Could you check a few things on this model? Use its own coordinates, in mm. A direction names the side the tool comes from. Give positions to 0.01 mm unless a question says otherwise; leave off trailing zeros. Order: outer loops, then holes, each group sorted by start corner. A loop starts at its lowest first (then second) coordinate and runs counter-clockwise, first axis right, second up.
(1) Imagine slicing it at B-B, the plane z = 15.25. Write out the boundary of the cut face in (x, y), then the cut area to 3 significant figures.
(2) On a 3-axis mill with a long thin cutter (end or side, diameter ignored), from which of +Z, -Z, +X, -X, +Y, -Y can I reach the whole of each face in a straight line? I mean faces 1 (the flat face through (85.725, -9, 5)), 2 (the flat face through (85.725, 9, 5)), 3 (the flat face through (95, 9, 5)). Say none if no direction works.
(3) If we mould it in two halves opening along Y, with no side actions, what happens to faces 4 (the cylindrical face through (95.19, 7.14, 2.46)), 5 (the cylindrical face through (42.452, 0.088, 15.16)), 6 (the flat face through (-85.725, 9, 5))? For each: released by +Y, released by -Y, zero draft, split by the parting line, or undercut.
(4) Imagine slicing it at C-C, the plane x = -49. Write out the boundary of the cut face in (y, z) (3 decimals).
(5) Will these pins go through, and if not, where does the flat tip stop? pin 1 (6 mm diameter, centred on y = -2.5, z = 5, fed in from -X); pin 2 (10 mm diameter, centred on y = 5.5, z = 17.5, fed in from -X); pin 3 (5 mm diameter, centred on x = -46.5, z = 5, fed in from -Y); pin 4 (3 mm diameter, centred on x = -93.66, y = -7.62, fed in from -Z).
(6) Imagine slicing it at A-A, the plane z = 7.75. Write out the boundary of the cut face in (x, y) (1 decimal).
(7) If I drill on probe 1 along X at (y, z) = (7.62, 1.45) (1 decimal); probe 2 along X at (y, z) = (-10, 1.75) (3 decimals); probe 3 along X at (y, z) = (0.25, 13.75), over which ranges is the centre line in solid material (lowest first)?
from build123d import *

# Parameters (mm, degrees)
F1_DEPTH = 9.525
F2_R     = 2.8
F3_DEPTH = 9.525
F4_R     = 2
F5_DEPTH = 12.7
F6_SIZE  = 1.27
F7_R     = 5.08
F8_R     = 2.8
F8_R_2   = 1.6
F9_DEPTH = 5


# Not quite as in the source:
# - a length typed as a fraction of an inch, garbled in the dataset ("3 / 203.2 mm" for 3/8 in), is restored


with BuildPart() as f1:
    # F0 (on Top) → F1 (new body)
    with BuildSketch(Plane.XY):
        Polygon((-85.725, -5.5000017), (85.725, -5.5000017), (85.725, -12.7), (101.6, -12.7), (101.6, -5.5000017), (101.6, 5.5000017), (101.6, 12.7), (85.725, 12.7), (85.725, 5.5000017), (-85.725, 5.5000017), (-85.725, 12.7), (-101.6, 12.7), (-101.6, 5.5000017), (-101.6, -5.5000017), (-101.6, -12.7), (-85.725, -12.7), align=None)
    extrude(amount=F1_DEPTH)

    # F2 (on face) → F3 (cut, through all)
    with BuildSketch(Plane.XY.offset(9.525)):
        with BuildLine():
            ThreePointArc((-93.6625, 4.82), (-91.6826010127, 5.6401010127), (-90.8625, 7.62))
            ThreePointArc((-90.8625, 7.62), (-91.6826010127, 9.5998989873), (-93.6625, 10.42))
            Line((-93.6625, 10.42), (-93.6625, 4.82))
        make_face()
        with BuildLine():
            ThreePointArc((-90.8625, -7.62), (-91.6826010127, -5.6401010127), (-93.6625, -4.82))
            Line((-93.6625, -4.82), (-93.6625, -10.42))
            ThreePointArc((-93.6625, -10.42), (-91.6826010127, -9.5998989873), (-90.8625, -7.62))
        make_face()
        with BuildLine():
            Line((-93.6625, -10.42), (-93.6625, -4.82))
            ThreePointArc((-93.6625, -4.82), (-96.4625, -7.62), (-93.6625, -10.42))
        make_face()
        with BuildLine():
            Line((-93.6625, 4.82), (-93.6625, 10.42))
            ThreePointArc((-93.6625, 10.42), (-96.4625, 7.62), (-93.6625, 4.82))
        make_face()
        with Locations((93.6625, 7.62)):
            Circle(F2_R)
        with Locations((93.6625, -7.62)):
            Circle(F2_R)
    extrude(amount=-F3_DEPTH, mode=Mode.SUBTRACT)

    # F4 (on face) → F5 (join)
    with BuildSketch(Plane.XY.offset(9.525)):
        with Locations((-44.45, 0)):
            Circle(F4_R)
        with Locations((44.45, 0)):
            Circle(F4_R)
    extrude(amount=F5_DEPTH)

    # F6
    f6_edges = [f1.edges().sort_by_distance(p)[0] for p in [
        (-46.45, 0, 22.225),
        (42.45, 0, 22.225),
    ]]
    chamfer(f6_edges, length=F6_SIZE)

    # F7
    f7_edges = [f1.edges().sort_by_distance(p)[0] for p in [
        (-101.6, 0, 9.525),
        (101.6, 0, 9.525),
    ]]
    fillet(f7_edges, radius=F7_R)

    # F8 (on face) → F9 (join)
    with BuildSketch(Plane(origin=(0, 0, 0), x_dir=(1, 0, 0), z_dir=(0, 0, -1))):
        with Locations((93.6625, 7.62)):
            Circle(F8_R)
        with Locations((93.6625, 7.62)):
            Circle(F8_R_2, mode=Mode.SUBTRACT)
        with Locations((93.6625, -7.62)):
            Circle(F8_R)
        with Locations((93.6625, -7.62)):
            Circle(F8_R_2, mode=Mode.SUBTRACT)
        with Locations((-93.6625, 7.62)):
            Circle(F8_R)
        with Locations((-93.6625, 7.62)):
            Circle(F8_R_2, mode=Mode.SUBTRACT)
        with Locations((-93.6625, -7.62)):
            Circle(F8_R)
        with Locations((-93.6625, -7.62)):
            Circle(F8_R_2, mode=Mode.SUBTRACT)
    extrude(amount=-F9_DEPTH)


solid = f1.part
Answer block:
1. outline: circle Ø4 at (-44.45, 0); circle Ø4 at (44.45, 0)
1. area: 25.1 mm2
2. face 1: +Z, -Z, -Y
2. face 2: +Z, -Z, +Y
2. face 3: +Z
3. face 4: undercut
3. face 5: split by the parting line
3. face 6: zero draft
4. outline: (-5.5, 0) - (5.5, 0) - (5.5, 9.525) - (-5.5, 9.525) - close
5. pin 1: stops at x = -101.6
5. pin 2: stops at x = -46.39
5. pin 3: stops at y = -5.5
5. pin 4: passes through
6. outline: (-100.4, -12.7) - (-85.7, -12.7) - (-85.7, -5.5) - (85.7, -5.5) - (85.7, -12.7) - (100.4, -12.7) - (100.4, 12.7) - (85.7, 12.7) - (85.7, 5.5) - (-85.7, 5.5) - (-85.7, 12.7) - (-100.4, 12.7) - close; hole circle Ø5.6 at (-93.7, -7.6); hole circle Ø5.6 at (-93.7, 7.6); hole circle Ø5.6 at (93.7, -7.6); hole circle Ø5.6 at (93.7, 7.6)
7. probe 1: x = -101.6 to -95.3, -92.1 to -85.7, 85.7 to 92.1, 95.3 to 101.6
7. probe 2: x = -101.6 to -85.725, 85.725 to 101.6
7. probe 3: x = -46.43 to -42.47, 42.47 to 46.43
